Read the model definition and answer for the solid it produces. Units are mm, in the model's axes. A direction names the side the tool comes from. Give positions to 0.01 mm unless a question says otherwise; leave off trailing zeros. Write each loop counter-clockwise with the first axis right and the second up, starting at its lowest first coordinate (ties: lowest second). Pieces come first, ordered by that corner, then holes. Notation, with made-up numbers: M 52.25,-38 L 60.25,-38 A20 ccw 60.25,-26 Z; hole C -40,41.25 d5. An arc over 180 degrees is marked long. Put each result on its own line as item: value.
Autodesk Inventor part; units mm, degrees
ref_plane "YZ Plane" through (0, 0, 0) normal (1, 0, 0) x (0, 1, 0)
ref_plane "XZ Plane" through (0, 0, 0) normal (0, 1, 0) x (-1, 0, 0)
ref_plane "XY Plane" through (0, 0, 0) normal (0, 0, 1) x (1, 0, 0)
sketch "Эскиз1" plane through (0, 0, 0) normal (0, 1, 0) x (-1, 0, 0)
  circle A0 centre (0, 0) radius 9
  dimension "d0" = 18
extrude "Выдавливание1" add sketch "Эскиз1" along normal blind 2
sketch "Эскиз5" plane through (0, 0, 0) normal (0, -1, 0) x (1, 0, 0)
  line L0 (5, -5) -> (-5, -5)
  line L1 (-5, -5) -> (-5, 5)
  line L2 (-5, 5) -> (5, 5)
  line L3 (5, 5) -> (5, -5)
  circle A0 centre (0, 0) radius 2
  dimension "d12" = 10
  dimension "d13" = 10
  dimension "d17" = 5
  dimension "d27" = 5
extrude "Выдавливание5" add sketch "Эскиз5" along normal blind 5
sketch "Эскиз6" plane through (-5, 0, -5) normal (-1, 0, 0) x (0, 0, 1)
  circle A0 centre (5, -2.5) radius 1.35
  line L0 (10, -5) -> (0, -5)
  line L1 (0, 0) -> (0, -5)
  point P0 (5, 0)
  point P1 (0, -2.5)
  dimension "d30" = 2.7
  dimension "d31" = 2.5
  dimension "d32" = 5
extrude "Выдавливание6" cut sketch "Эскиз6" against normal blind 15.75
fillet "Сопряжение1" radius 5 4 edges at (5, -2.5, 5) (-5, -2.5, 5) (-5, -2.5, -5) (5, -2.5, -5)
sketch "Эскиз8" plane through (0, 0, 0) normal (0, -1, 0) x (1, 0, 0)
  point P0 (0, 0)
sketch "Эскиз9" plane through (0, 2, 0) normal (0, 1, 0) x (1, 0, 0)
  circle A0 centre (0, 0) radius 2.15
  dimension "d44" = 4.3
extrude "Выдавливание8" cut sketch "Эскиз9" against normal blind 10
sketch "Эскиз11" plane through (0, 2, 0) normal (0, 1, 0) x (1, 0, 0)
  circle A0 centre (0, 0) radius 5
  dimension "d47" = 10
extrude "Выдавливание9" add sketch "Эскиз11" along normal blind 5.2
sketch "Эскиз12" plane through (0, 7.2, 0) normal (0, 1, 0) x (1, 0, 0)
  circle A0 centre (0, 0) radius 9
  dimension "d50" = 18
extrude "Выдавливание10" add sketch "Эскиз12" along normal blind 2
sketch "Эскиз13" plane through (0, 9.2, 0) normal (0, 1, 0) x (1, 0, 0)
  circle A0 centre (0, 0) radius 2
  dimension "d53" = 4
extrude "Выдавливание11" cut sketch "Эскиз13" against normal blind 17.75
sketch "Эскиз14" plane through (0, 9.2, 0) normal (0, 1, 0) x (1, 0, 0)
  circle A0 centre (0, 0) radius 2.5
  dimension "d56" = 5
extrude "Выдавливание12" add sketch "Эскиз14" along normal blind 1.5
sketch "Эскиз15" plane through (0, 10.7, 0) normal (0, 1, 0) x (1, 0, 0)
  circle A0 centre (0, 0) radius 2
  dimension "d59" = 4
extrude "Выдавливание13" cut sketch "Эскиз15" against normal blind 33.5
properties part number "koleso_rig"
(1) Straight lines are drawn through the part: line 1 along Y through (x, z) = (4.35, 0); line 2 along Z through (x, y) = (0, -3); line 3 along Y through (x, z) = (-0.5, -7). For each, find the intervals that lie inside material, in ascending order. Write a range as from..to.
Result:
line 1: y = -5..-3.85, -1.15..9.2
line 2: z = -5..-2.15, 2.15..5
line 3: y = 0..2, 7.2..9.2
(2) Section D-D on z = 0 is taken. Give the number of separate pieces and of enclosed holes in the cut face, and give its area (3 significant figures).
Result:
separate pieces: 4
enclosed holes: 0
area: 101 mm²
(3) Given pin 1 Ø4 at (x, z) = (6, -0.5) entering from +Y; pin 2 Ø4.5 at (y, z) = (-2.5, 0) entering from -X; pin 3 Ø2 at (x, z) = (1, -0.5) entering from -Y, each flat-ended and moving along its own axis, determine where each tip first touches the part or whether it passes through.
Result:
pin 1: stops at y = 9.2
pin 2: stops at x = -5
pin 3: stops at y = 2
(4) Section A-A on x = 0 is taken. Determine the outline of the cut face in (y, z).
Result:
outline: M -5,-5 L 0,-5 L 0,-9 L 2,-9 L 2,-5 L 7.2,-5 L 7.2,-9 L 9.2,-9 L 9.2,-2.5 L 10.7,-2.5 L 10.7,-2 L 2,-2 L 2,-2.15 L -5,-2.15 Z; M -5,2.15 L 2,2.15 L 2,2 L 10.7,2 L 10.7,2.5 L 9.2,2.5 L 9.2,9 L 7.2,9 L 7.2,5 L 2,5 L 2,9 L 0,9 L 0,5 L -5,5 Z
(5) Section C-C on z = -5.25 is taken. Determine the outline of the cut face in (x, y).
Result:
outline: M -7.31,0 L 7.31,0 L 7.31,2 L -7.31,2 Z; M -7.31,7.2 L 7.31,7.2 L 7.31,9.2 L -7.31,9.2 Z
(6) For a pull along Y with two mould halves and no side action, classify faces 1 (the face through (2.2, -5, -1)), 2 (the face through (-3.36, -3.82, -0.29)), 3 (the face through (0, 6, 2)) as +Y half, -Y half, draft (parallel to the pull), parting line (faces both ways), or undercut.
Result:
face 1: -Y half
face 2: undercut
face 3: draft
(7) Which of the six approach directions +Z, -Z, +X, -X, +Y, -Y give full straight-line access (tool end or side, diameter ignored) to faces 4 (the face through (-1.585, -1.451, -1.453)), 5 (the face through (3.313, -3.017, 1.247)), 6 (the face through (4, 7.2, 4)), 7 (the face through (-1.172, 8.186, 8.923)), 8 (the face through (-0.54, 9.94, -2.44))?
Result:
face 4: -Y
face 5: +X, -X
face 6: none
face 7: +Y, -Y
face 8: +Y
(8) Section B-B on y = -2.5 is taken. Determine the outline of the cut face in (x, z), and give its area (3 significant figures).
Result:
outline: M -4.81,-1.35 A5 ccw 4.81,-1.35 L 1.67,-1.35 A2.15 cw -1.67,-1.35 Z; M -4.81,1.35 L -1.67,1.35 A2.15 cw 1.67,1.35 L 4.81,1.35 A5 ccw Z
area: 48.1 mm²
